For this review, use the dimensioned drawing (mm, ordinates from the lowest corner) and the shaded views. A direction names the side the tool comes from. Give positions to 0.01 mm unless a question says otherwise; leave off trailing zeros. Order: outer loops, then holes, each group sorted by start corner. A loop starts at its lowest first (then second) coordinate and runs counter-clockwise, first axis right, second up. Notation, with made-up numbers: (50.25, -19) - (64.25, -19) arc R31 ccw to (64.25, 20) - close; hole circle Ø9 at (6, 78). An arc over 180 degrees is marked (long way). Use a Markdown table: item, result. Add a question column.
1) We need section A-A on y = 43. Write out the cut boundary in (x, z).
2) We need section C-C on z = 11.5. Write out the cut boundary in (x, y).
3) Machinability: for the marked faces 1 and 2, which of the approach directions +Z, -Z, +X, -X, +Y, -Y give a long, thin tool a straight path to every point of the face, cutting with its end or side? Answer none if there is none.
4) We need section B-B on x = 38.5. Write out the cut boundary in (y, z).
5) Wall thickness on L1, parallel to Y at x = 39.5, z = 2; L2, parallel to X at y = 52.5, z = 41.5; L3, parallel to X at y = 58, z = 25: over which ranges is each line inside the solid? List them lowest first.
6) Mouldability with a two-part tool opening along X and no side actions: class the marked faces 3, 4 and 5 as released by +X, released by -X, zero draft, split by the parting line, or undercut.
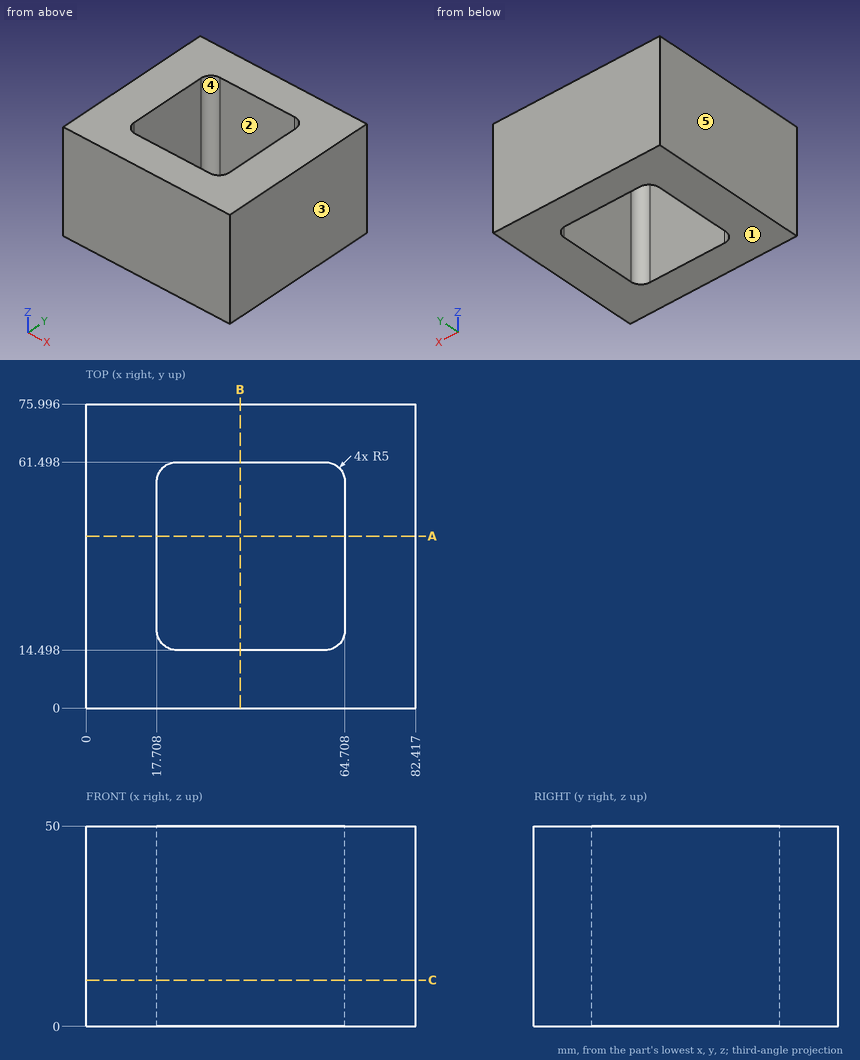
Checked values:
| question | item | result |
|---|---|---|
| 1 | outline | (0, 0) - (17.71, 0) - (17.71, 50) - (0, 50) - close; (64.71, 0) - (82.42, 0) - (82.42, 50) - (64.71, 50) - close |
| 2 | outline | (0, 0) - (82.42, 0) - (82.42, 76) - (0, 76) - close; hole (17.71, 19.5) arc R5 ccw to (22.71, 14.5) - (59.71, 14.5) arc R5 ccw to (64.71, 19.5) - (64.71, 56.5) arc R5 ccw to (59.71, 61.5) - (22.71, 61.5) arc R5 ccw to (17.71, 56.5) - close |
| 3 | face 1 | -Z, +X, -X, +Y, -Y |
| 3 | face 2 | +Z, -Z |
| 4 | outline | (0, 0) - (14.5, 0) - (14.5, 50) - (0, 50) - close; (61.5, 0) - (76, 0) - (76, 50) - (61.5, 50) - close |
| 5 | L1 | 0 to 14.5, 61.5 to 76 |
| 5 | L2 | 0 to 17.71, 64.71 to 82.42 |
| 5 | L3 | 0 to 17.94, 64.48 to 82.42 |
| 6 | face 3 | released by +X |
| 6 | face 4 | undercut |
| 6 | face 5 | released by -X |
